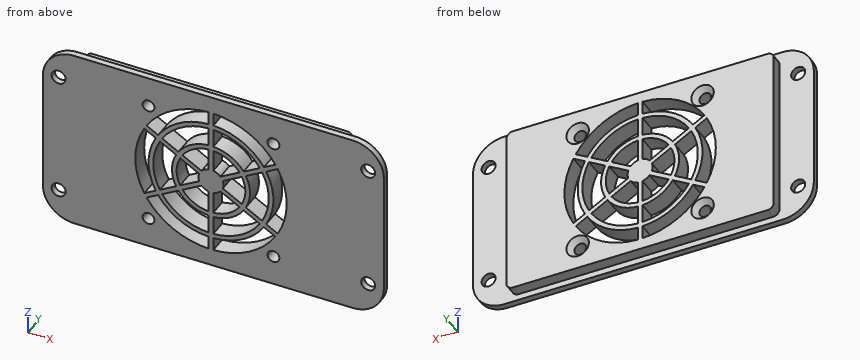
Autodesk Fusion 360 part; units mm, degrees
sketch "Sketch1" plane through (0, 0, 0) normal (0, 1, 0) x (1, 0, 0)
  line L0 (0, 0) -> (85.6, 0)
  line L1 (85.6, 0) -> (85.6, 55.5)
  line L2 (85.6, 55.5) -> (0, 55.5)
  line L3 (0, 55.5) -> (0, 0)
  line L4 (0, 55.5) -> (85.6, 0) construction
  line L5 (0, 0) -> (85.6, 55.5) construction
  line L6 (62.8, 47.75) -> (22.8, 47.75) construction
  line L7 (22.8, 47.75) -> (22.8, 7.75) construction
  line L8 (22.8, 7.75) -> (62.8, 7.75) construction
  line L9 (62.8, 7.75) -> (62.8, 47.75) construction
  line L10 (62.8, 47.75) -> (22.8, 7.75) construction
  line L11 (22.8, 47.75) -> (62.8, 7.75) construction
  circle A0 centre (62.8, 47.75) radius 1.9
  circle A1 centre (62.8, 7.75) radius 1.9
  circle A2 centre (22.8, 7.75) radius 1.9
  circle A3 centre (22.8, 47.75) radius 1.9
  line L12 (68.05, 2.5) -> (17.55, 2.5) construction
  line L13 (17.55, 2.5) -> (17.55, 53) construction
  line L14 (17.55, 53) -> (68.05, 53) construction
  line L15 (68.05, 53) -> (68.05, 2.5) construction
  line L16 (68.05, 2.5) -> (17.55, 53) construction
  line L17 (17.55, 2.5) -> (68.05, 53) construction
  circle A4 centre (42.8, 27.75) radius 24.25
  line L18 (43.55, 53) -> (42.05, 53) construction
  line L19 (42.05, 53) -> (42.05, 27.75)
  line L20 (42.05, 27.75) -> (43.55, 27.75)
  line L21 (43.55, 27.75) -> (43.55, 53)
  line L22 (43.175, 28.3995) -> (21.3079, 41.0245)
  line L23 (20.5579, 39.7255) -> (42.425, 27.1005)
  line L24 (42.425, 28.3995) -> (20.5579, 15.7745)
  line L25 (21.3079, 14.4755) -> (43.175, 27.1005)
  line L26 (42.05, 27.75) -> (42.05, 2.5)
  line L27 (43.55, 2.5) -> (43.55, 27.75)
  line L28 (42.425, 27.1005) -> (64.2921, 14.4755)
  line L29 (65.0421, 15.7745) -> (43.175, 28.3995)
  line L30 (43.175, 27.1005) -> (65.0421, 39.7255)
  line L31 (64.2921, 41.0245) -> (42.425, 28.3995)
  circle A5 centre (42.8, 27.75) radius 20
  circle A6 centre (42.8, 27.75) radius 18.5
  circle A7 centre (42.8, 27.75) radius 12.5
  circle A8 centre (42.8, 27.75) radius 11
  circle A9 centre (42.8, 27.75) radius 4
  line L32 (85.6, 7.25) -> (95.4, 7.25) construction
  circle A10 centre (93.15, 7.25) radius 2.25
  line L33 (93.15, 7.25) -> (93.15, 9.5) construction
  line L34 (93.15, 9.5) -> (93.15, 45) construction
  circle A11 centre (93.15, 47.25) radius 2.25
  line L35 (93.15, 47.25) -> (93.15, 45) construction
  line L36 (85.6, 0) -> (93.15, 0) construction
  line L37 (93.15, 0) -> (93.15, 7.25) construction
  line L38 (85.6, 7.25) -> (0, 7.25) construction
  line L39 (0, 7.25) -> (-6, 7.25) construction
  line L40 (-6, 7.25) -> (-6, 47.25) construction
  line L41 (93.15, 47.25) -> (-6, 47.25) construction
  circle A12 centre (-6, 47.25) radius 2.25
  circle A13 centre (-6, 7.25) radius 2.25
  line L42 (-11, 57.5) -> (98.15, 57.5)
  line L43 (98.15, 57.5) -> (98.15, -2)
  line L44 (98.15, -2) -> (-11, -2)
  line L45 (-11, -2) -> (-11, 57.5)
  point P0 (42.8, 27.75)
  point P1 (42.8, 27.75)
  dimension "d1" = 85.6
  dimension "d2" = 55.5
  dimension "d3" = 40
  dimension "d4" = 40
  dimension "d5" = 3.8
  dimension "d6" = 3.8
  dimension "d7" = 3.8
  dimension "d8" = 3.8
  dimension "d9" = 50.5
  dimension "d10" = 50.5
  dimension "d11" = 48.5
  dimension "d12" = 1.5
  dimension "d14" = 360
  dimension "d15" = -1.5
  dimension "d16" = 25
  dimension "d17" = -1.5
  dimension "d18" = 8
  dimension "d19" = 9.8
  dimension "d20" = 4.5
  dimension "d21" = 35.5
  dimension "d22" = 4.5
  dimension "d23" = 7.25
  dimension "d24" = 6
  dimension "d25" = 4.5
  dimension "d26" = 4.5
  dimension "d27" = 5
  dimension "d28" = 5
  dimension "d29" = 2
  dimension "d30" = 2
extrude "Extrude1" add sketch "Sketch1" along normal blind 3.6 and the other way blind 2 contours L0 L1 L2 L3 | A4 L30 L31 A5 | A4 L28 L29 A5 | L29 L30 A5 A6 | L30 L31 A5 A6 | L28 L29 A5 A6 | A4 L19 L21 A5 | L21 L31 A5 A6 | L30 L31 A6 A7 | A4 L26 L27 A5 | L27 L28 A5 A6 | L28 L29 A6 A7 | L19 L21 A5 A6 | L29 L30 A7 A8 | L30 L31 A7 A8 | L26 L27 A5 A6 | L28 L29 A7 A8 | A4 L22 L23 A5 | L19 L22 A5 A6 | L19 L21 A6 A7 | L21 L31 A7 A8 | L30 L31 A8 A9 | A4 L24 L25 A5 | L25 L26 A5 A6 | L26 L27 A6 A7 | L27 L28 A7 A8 | L28 L29 A8 A9 | L22 L23 A5 A6 | L19 L21 A7 A8 | L29 L30 A9 | L21 L29 L30 L31 A9 | L24 L25 A5 A6 | L26 L27 A7 A8 | L27 L28 L29 L30 A9 | L23 L24 A5 A6 | L22 L23 A6 A7 | L19 L22 A7 A8 | L19 L21 A8 A9 | L21 L31 A9 | L21 L27 L29 L30 | L24 L25 A6 A7 | L25 L26 A7 A8 | L26 L27 A8 A9 | L27 L28 A9 | L22 L23 A7 A8 | L19 L21 L22 L31 A9 | L21 L22 L29 L31 | L19 L20 L21 L22 L24 L29 L31 | L20 L23 L25 L26 L27 L28 L30 | L25 L27 L28 L30 | L24 L25 A7 A8 | L25 L26 L27 L28 A9 | L23 L24 A7 A8 | L22 L23 A8 A9 | L19 L22 A9 | L19 L22 L24 L31 | L24 L25 A8 A9 | L25 L26 A9 | L23 L25 L26 L28 | L19 L22 L23 L24 A9 | L19 L23 L24 L26 | L23 L24 L25 L26 A9 | L23 L24 A9
extrude "Extrude2" add sketch "Sketch1" against normal blind 2 contours L42 L43 L44 L45
fillet "Fillet1" radius 10 4 edges at (98.15, -1, -57.5) (98.15, -1, 2) (-11, -1, 2) (-11, -1, -57.5)
fillet "Fillet2" radius 2 4 edges at (0, 1.8, 0) (85.6, 1.8, 0) (85.6, 1.8, -55.5) (0, 1.8, -55.5)
chamfer "Chamfer1" distance 1.7 angle 45 4 edges at (21.0286, 3.6, -48.4371) (61.0286, 3.6, -48.4371) (61.0286, 3.6, -8.4371) (21.0286, 3.6, -8.4371)
Read the model definition and answer for the solid it produces. Units are mm, in the model's axes. Give positions to 0.01 mm unless a question says otherwise; leave off trailing zeros. Write each loop counter-clockwise with the first axis right and the second up, starting at its lowest first coordinate (ties: lowest second). Pieces come first, ordered by that corner, then holes. Notation, with made-up numbers: (50, 50.5) -> (61, 50.5) arc R9 cw to (61, 63.5) -> close; hole circle Ø2 at (15, 52.25). An arc over 180 degrees is marked (long way). Answer in a Markdown table with one row per item.
1) Section A-A on x = 12 is taken. Give the vertices of the cut face in (y, z).
Results list:
| item | result |
|---|---|
| outline | (-2, -57.5) -> (0, -57.5) -> (0, -55.5) -> (3.6, -55.5) -> (3.6, 0) -> (0, 0) -> (0, 2) -> (-2, 2) -> close |
2) Straight lines are drawn through the part: line 1 (Z direction, x = 93.15, y = -0.95); line 2 (X direction, y = -1.55, z = -11.5); line 3 (Z direction, x = 29.5, y = 1.55). For each, find the intervals that lie inside material, in ascending order. Write a range as [from, to].
Results list:
| item | result |
|---|---|
| line 1 | [-56.16, -49.5], [-45, -9.5], [-5, 0.66] |
| line 2 | [-11, 24.8], [31.14, 33.96], [42.05, 43.55], [51.64, 54.46], [60.8, 98.15] |
| line 3 | [-55.5, -48.03], [-42.69, -40.61], [-36.29, -34.56], [-20.94, -19.21], [-14.89, -12.81], [-7.47, 0] |
3) Section B-B on x = 93.15 is taken. Give the vertices of the cut face in (y, z).
Results list:
| item | result |
|---|---|
| outline | (-2, -56.16) -> (0, -56.16) -> (0, -49.5) -> (-2, -49.5) -> close; (-2, -45) -> (0, -45) -> (0, -9.5) -> (-2, -9.5) -> close; (-2, -5) -> (0, -5) -> (0, 0.66) -> (-2, 0.66) -> close |
4) Each of these flat-tipped pins is pushed along its axis until it touches: pin 1 Ø2.5 at (x, z) = (62.8, -47.75) entering from +Y; pin 2 Ø12 at (x, z) = (20, -35) entering from +Y; pin 3 Ø1.1 at (x, y) = (29, 2) entering from +Z; pin 4 Ø2 at (y, z) = (1.5, -49.5) entering from -X. Where does it stop, or does it pass through?
Results list:
| item | result |
|---|---|
| pin 1 | through |
| pin 2 | y = 3.6 |
| pin 3 | z = 0 |
| pin 4 | x = 0 |
